```python
from build123d import *

# Parameters (mm, degrees)
SKETCH_1_R      = 3.5
SKETCH_1_R_2    = 1.5
EXTRUDE_2_DEPTH = 30
SKETCH_3_R      = 0.45
EXTRUDE_4_DEPTH = 1.5


with BuildPart() as part:
    # 草图1 → 凸台-拉伸2 (new body)
    with BuildSketch(Plane(origin=(0, 0, 0), x_dir=(1, 0, 0), z_dir=(0, 1, 0))):
        with Locations(Location((0, 0, 0), (0, 0, 270))):
            Circle(SKETCH_1_R)
        with Locations(Location((0, 0, 0), (0, 0, 270))):
            Circle(SKETCH_1_R_2, mode=Mode.SUBTRACT)
    extrude(amount=EXTRUDE_2_DEPTH)

    # 草图3 → 凸台-拉伸4 (add)
    with BuildSketch(Plane(origin=(0, 30, 0), x_dir=(1, 0, 0), z_dir=(0, 1, 0))):
        with Locations(Location((0, 2.5, 0), (0, 0, 270))):
            Circle(SKETCH_3_R)
        with Locations(Location((2.5, 0, 0), (0, 0, 270))):
            Circle(SKETCH_3_R)
        with Locations(Location((0, -2.5, 0), (0, 0, 270))):
            Circle(SKETCH_3_R)
        with Locations(Location((-2.5, 0, 0), (0, 0, 270))):
            Circle(SKETCH_3_R)
    extrude(amount=EXTRUDE_4_DEPTH)


solid = part.part
```
Can you work these out from the model? Positions are in its coordinate system, mm. A direction names the side the tool comes from. Coordinates: 2 decimals unless noted, no trailing zeros. Loops run counter-clockwise (first coordinate to the right, second up) from the corner with the lowest first, then second, coordinate; pieces in that order, holes last. Notation, with made-up numbers: (-9, -4) - (35, -4) arc R27 cw to (35, 31) - close; hole circle Ø11 at (83.5, -40). An arc over 180 degrees is marked (long way). Use a Markdown table: item, result.
Item 1: I want a section at C-C on y = 27.5. Please give me the cut outline in (x, z).
Numbers:
| item | result |
|---|---|
| outline | circle Ø7 at (0, 0); hole circle Ø3 at (0, 0) |
Item 2: I want a section at A-A on x = 0. Please give me the cut outline in (y, z), and give its area (3 significant figures).
Numbers:
| item | result |
|---|---|
| outline | (0, -3.5) - (30, -3.5) - (30, -2.95) - (31.5, -2.95) - (31.5, -2.05) - (30, -2.05) - (30, -1.5) - (0, -1.5) - close; (0, 1.5) - (30, 1.5) - (30, 2.05) - (31.5, 2.05) - (31.5, 2.95) - (30, 2.95) - (30, 3.5) - (0, 3.5) - close |
| area | 123 mm2 |
Item 3: For faces 4 (the face through (0.02, 30.74, -2.95)), 5 (the face through (0, 0, 2)), which set-ups out of +Z, -Z, +X, -X, +Y, -Y let a thin tool reach every point of the face, with its end or its side?
Numbers:
| item | result |
|---|---|
| face 4 | +Y |
| face 5 | +Z, -Z, +X, -X, -Y |
Item 4: I want a section at D-D on x = 2.5. Please give me the cut outline in (y, z), and give its area (3 significant figures).
Numbers:
| item | result |
|---|---|
| outline | (0, -2.45) - (30, -2.45) - (30, -0.45) - (31.5, -0.45) - (31.5, 0.45) - (30, 0.45) - (30, 2.45) - (0, 2.45) - close |
| area | 148 mm2 |
Item 5: I want a section at B-B on z = 0.75. Please give me the cut outline in (x, y), and give its area (3 significant figures).
Numbers:
| item | result |
|---|---|
| outline | (-3.42, 0) - (-1.3, 0) - (-1.3, 30) - (-3.42, 30) - close; (1.3, 0) - (3.42, 0) - (3.42, 30) - (1.3, 30) - close |
| area | 127 mm2 |
Item 6: We'd pull the mould along X, two halves only. Please class faces 1 (the face through (-2.94, 30.74, -0.1)), 2 (the face through (0.02, 30.74, 2.05)), 3 (the face through (0, 31.5, -2.5)): released by +X, released by -X, zero draft, split by the parting line, or undercut.
Numbers:
| item | result |
|---|---|
| face 1 | undercut |
| face 2 | split by the parting line |
| face 3 | zero draft |
Item 7: Will this pin go through, and if not, where does the flat tip stop? pin 1 (1 mm diameter, centred on y = 3.5, z = 1, fed in from +X).
Numbers:
| item | result |
|---|---|
| pin 1 | stops at x = 3.46 |
Item 8: If I drill on probe 1 along X at (y, z) = (21, 0); probe 2 along Y at (x, z) = (1.5, -0.5); probe 3 along Z at (x, y) = (-1.25, 4.5), over which ranges is the centre line in solid material (lowest first)? Write a range as from..to.
Numbers:
| item | result |
|---|---|
| probe 1 | x = -3.5..-1.5, 1.5..3.5 |
| probe 2 | y = 0..30 |
| probe 3 | z = -3.27..-0.83, 0.83..3.27 |
